The drawing under review shows one solid part. Ordinate dimensions are in mm from its lowest x, y, z. A direction names the side the tool comes from. Coordinates: 2 decimals unless noted, no trailing zeros. Write each loop counter-clockwise with the first axis right and the second up, starting at its lowest first coordinate (ties: lowest second). Pieces come first, ordered by that corner, then holes.
Q1. Add section C-C, the plane x = 44. Give the boundary of the cut face in (y, z).
Q2. Add section A-A, the plane x = 13.5. Give the boundary of the cut face in (y, z).
Q3. The part is to be moulded in two halves that separate along Z. For the marked faces 1, 2, 3 and 4, say which applies: +Z half, -Z half, draft (parallel to the pull), parting line (faces both ways), or undercut.
Q4. Machinability: for the marked faces 5, 6 and 7, which of the approach directions +Z, -Z, +X, -X, +Y, -Y give a long, thin tool a straight path to every point of the face, cutting with its end or side? Answer none if there is none.
Q5. To check wall thickness, follow probe 1 along Z at (x, y) = (13.5, 16.25); probe 2 along Z at (x, y) = (14.5, 22.75); probe 3 along X at (y, z) = (11.25, 18.75). State the ranges of each line that lie inside material, in increasing order.
Q6. Add section B-B, the plane y = 12.5. Give the boundary of the cut face in (x, z).
Q7. Add section D-D, the plane z = 18.5. Give the boundary of the cut face in (x, y).
Q8. Clearance check with flat-ended pins moving along their axes: pin 1 Ø1.9 at (y, z) = (14.5, 16) entering from +X; pin 2 Ø1.9 at (y, z) = (12, 20.5) entering from +X; pin 3 Ø6.5 at (x, z) = (12.5, 18.5) entering from -Y. State where each tip first meets the part, or that it passes through.
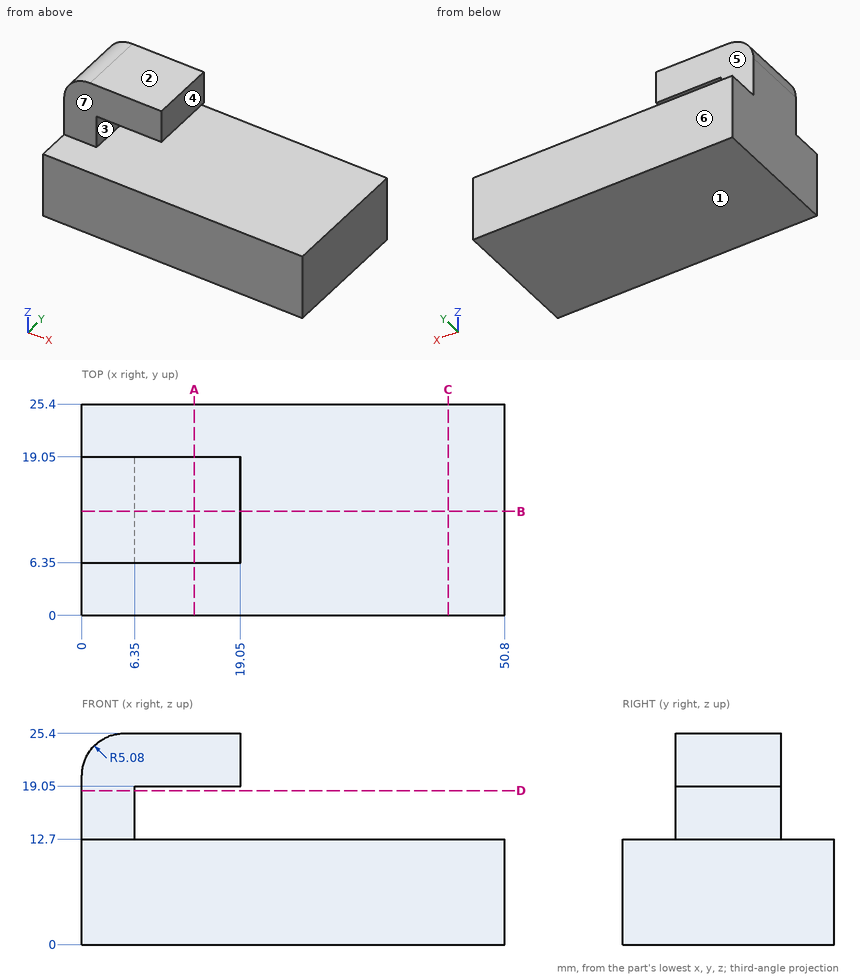
Here are the results:
1. outline: (0, 0) - (25.4, 0) - (25.4, 12.7) - (0, 12.7) - close
2. outline: (0, 0) - (25.4, 0) - (25.4, 12.7) - (0, 12.7) - close; (6.35, 19.05) - (19.05, 19.05) - (19.05, 25.4) - (6.35, 25.4) - close
3. face 1: -Z half
3. face 2: +Z half
3. face 3: undercut
3. face 4: draft
4. face 5: +Z, +X, -X, +Y
4. face 6: +Z, -Z, +X, -X, +Y
4. face 7: +Z, +X, -X, -Y
5. probe 1: z = 0 to 12.7, 19.05 to 25.4
5. probe 2: z = 0 to 12.7
5. probe 3: x = 0 to 6.35
6. outline: (0, 0) - (50.8, 0) - (50.8, 12.7) - (6.35, 12.7) - (6.35, 19.05) - (19.05, 19.05) - (19.05, 25.4) - (5.08, 25.4) arc R5.08 ccw to (0, 20.32) - close
7. outline: (0, 6.35) - (6.35, 6.35) - (6.35, 19.05) - (0, 19.05) - close
8. pin 1: stops at x = 6.35
8. pin 2: stops at x = 19.05
8. pin 3: stops at y = 6.35
